from build123d import *

# Parameters (mm, degrees)
F1_DEPTH = 12.7
F4_DEPTH = 6.35
F6_D     = 2.2606
F6_DEPTH = 12.7
F6_TIP   = 0.6791527577
F7_R     = 2.54
F8_DEPTH = 3.175


with BuildPart() as f1:
    # F0 (on Top) → F1 (new body)
    with BuildSketch(Plane.XY):
        Polygon((-101.6, 127), (101.6, 127), (114.3, 114.3), (114.3, -114.3), (101.6, -114.3), (101.6, -139.7), (114.3, -139.7), (127, -139.7), (127, -114.3), (127, 114.3), (127, 139.7), (101.6, 139.7), (-101.6, 139.7), (-127, 139.7), (-127, 114.3), (-127, -114.3), (-127, -139.7), (-114.3, -139.7), (-101.6, -139.7), (-101.6, -114.3), (-114.3, -114.3), (-114.3, 114.3), align=None)
    extrude(amount=F1_DEPTH)

    # F3 (on face) → F4 (cut)
    with BuildSketch(Plane(origin=(0, 0, 0), x_dir=(1, 0, 0), z_dir=(0, 0, -1))):
        Polygon((-117.475, 121.500738686), (-111.125, 121.500738686), (-107.95, 127), (-111.125, 132.499261314), (-117.475, 132.499261314), (-120.65, 127), align=None)
        Polygon((-107.95, -127), (-111.125, -121.500738686), (-117.475, -121.500738686), (-120.65, -127), (-117.475, -132.499261314), (-111.125, -132.499261314), align=None)
        Polygon((120.65, -127), (117.475, -121.500738686), (111.125, -121.500738686), (107.95, -127), (111.125, -132.499261314), (117.475, -132.499261314), align=None)
        Polygon((120.65, 127), (117.475, 132.499261314), (111.125, 132.499261314), (107.95, 127), (111.125, 121.500738686), (117.475, 121.500738686), align=None)
    extrude(amount=-F4_DEPTH, mode=Mode.SUBTRACT)

    # F6
    with Locations(Plane.XY.offset(12.7)):
        with Locations((-114.3, 127), (-114.3, -127), (114.3, -127), (114.3, 127)):
            Hole(F6_D / 2, depth=F6_DEPTH)
            with Locations((0, 0, -(F6_DEPTH + F6_TIP / 2))):  # 118° drill point
                Cone(0, F6_D / 2, F6_TIP, mode=Mode.SUBTRACT)

    # F7 (on face) → F8 (cut)
    with BuildSketch(Plane.XY.offset(12.7)):
        with Locations((-114.3, 127)):
            Circle(F7_R)
        with Locations((114.3, 127)):
            Circle(F7_R)
        with Locations((114.3, -127)):
            Circle(F7_R)
        with Locations((-114.3, -127)):
            Circle(F7_R)
    extrude(amount=-F8_DEPTH, mode=Mode.SUBTRACT)


solid = f1.part
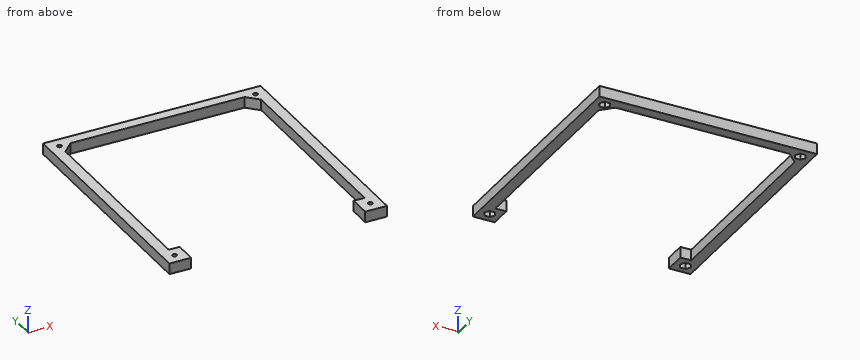
Source: CAD feature listing. Evaluate the final solid. Frame: model axes, mm. Coordinates: 2 decimals unless noted, no trailing zeros. Order: outer loops, then holes, each group sorted by start corner. A loop starts at its lowest first (then second) coordinate and runs counter-clockwise, first axis right, second up. Notation, with made-up numbers: M 10,55 L 17,55 A19 cw 17,60 Z; hole C -35.5,49 d4. An arc over 180 degrees is marked long. Write each question's results on one line, items separated by ' | '. Start each with the question number.
1. Section A-A, the plane y = -64.5. Return the cut outline in (x, z).
2. Section C-C, the plane x = -41.5. Return the cut outline in (y, z).
3. Pin query (flat end, axial travel): pin 1 (5.5 mm diameter, centred on x = 115, y = -128.5, fed in from -Z); pin 2 (4 mm diameter, centred on x = -68.5, z = 6, fed in from -Y); pin 3 (3 mm diameter, centred on x = 114.3, y = -127, fed in from -Z). Return the tip coordinate at first contact, or that it passes through.
4. Material intervals for L1, parallel to X at y = 105, z = 1.5; L2, parallel to Y at x = -31, z = 4.25; L3, parallel to Y at x = 107, z = 2, sorted ascending.
5. Section B-B, the plane z = 2.75. State how many separate pieces and enclosed holes the cut face has, then the cut area to 3 significant figures.
Solution:
1) outline: M -127,0 L -114.3,0 L -114.3,12.7 L -127,12.7 Z; M 114.3,0 L 127,0 L 127,12.7 L 114.3,12.7 Z
2) outline: M 127,0 L 139.7,0 L 139.7,12.7 L 127,12.7 Z
3) pin 1: z = 6.35 | pin 2: y = 127 | pin 3: z = 6.35
4) L1: -127 to -114.3, 114.3 to 127 | L2: 127 to 139.7 | L3: -139.7 to -114.3, 121.6 to 139.7
5) separate pieces: 1 | enclosed holes: 4 | area: 10,400 mm²
